For this review, use the dimensioned drawing (mm, ordinates from the lowest corner) and the shaded views. Give positions to 0.01 mm unless a question says otherwise; leave off trailing zeros. Order: outer loops, then holes, each group sorted by start corner. A loop starts at its lowest first (then second) coordinate and runs counter-clockwise, first axis right, second up. Notation, with made-up numbers: (5, 77.5) - (23, 77.5) arc R25 cw to (23, 111.5) - close; hole circle Ø4 at (31.5, 43.5). An arc over 180 degrees is marked (long way). Use a Markdown table: item, result. Add a question column.
1) We need section C-C on z = 16. Write out the cut boundary in (x, y), then the cut area to 3 significant figures.
2) Mouldability with a two-part tool opening along Y and no side actions: class the marked faces 1, 2 and 3 as released by +Y, released by -Y, zero draft, split by the parting line, or undercut.
3) Clearance check with flat-ended pins moving along their axes: P1, Ø3, axis at y = 29, z = 45, coming from the -X side; P2, Ø3, axis at y = 40, z = 16, coming from the -X side; P3, Ø12, axis at x = 164, y = 180, coming from the +Z side. State where each tip first meets the part, or that it passes through.
4) We need section A-A on x = 101.6. Write out the cut boundary in (y, z).
5) We need section B-B on z = 34.5. Write out the cut boundary in (x, y).
6) Wall thickness on L1, parallel to X at y = 101, z = 25; L2, parallel to Y at x = 101.6, z = 28; L3, parallel to X at y = 80, z = 44: over which ranges is each line inside the solid? List them lowest first.
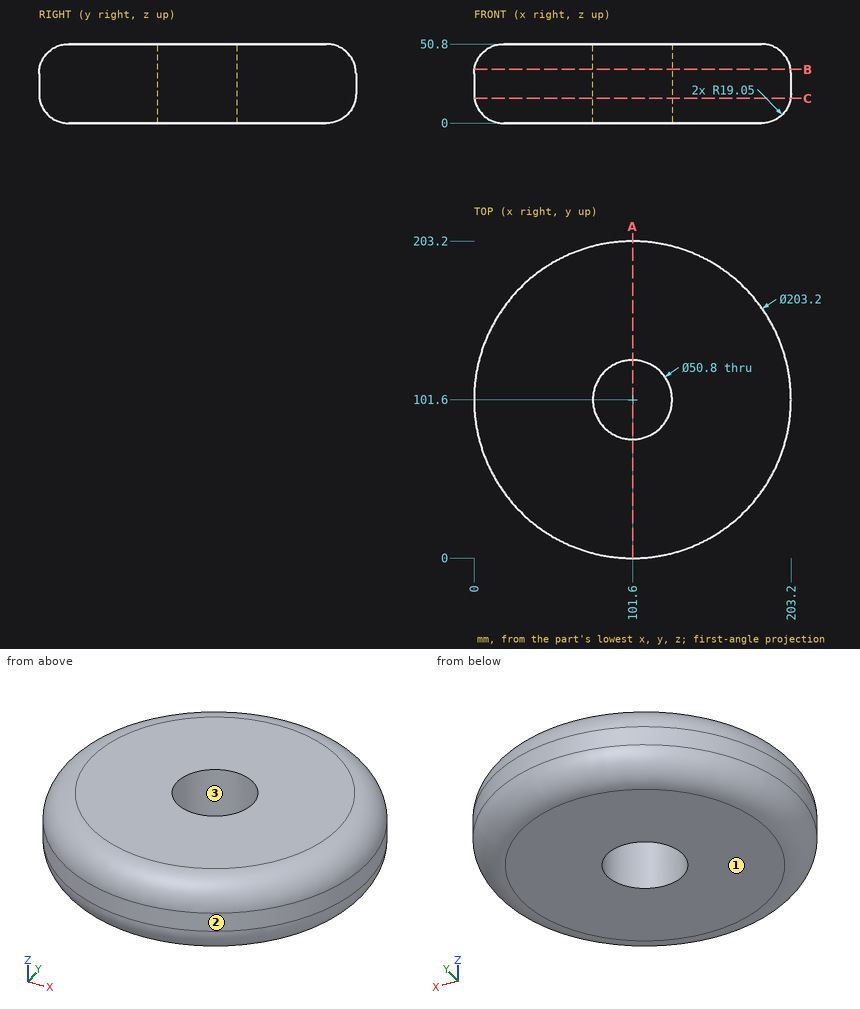
Checked values:
| question | item | result |
|---|---|---|
| 1 | outline | circle Ø202.71 at (101.6, 101.6); hole circle Ø50.8 at (101.6, 101.6) |
| 1 | area | 30,200 mm² |
| 2 | face 1 | zero draft |
| 2 | face 2 | split by the parting line |
| 2 | face 3 | undercut |
| 3 | P1 | x = 35.81 |
| 3 | P2 | x = 19.95 |
| 3 | P3 | z = 46.82 |
| 4 | outline | (0, 19.05) arc R19.05 ccw to (19.05, 0) - (76.2, 0) - (76.2, 50.8) - (19.05, 50.8) arc R19.05 ccw to (0, 31.75) - close; (127, 0) - (184.15, 0) arc R19.05 ccw to (203.2, 19.05) - (203.2, 31.75) arc R19.05 ccw to (184.15, 50.8) - (127, 50.8) - close |
| 5 | outline | circle Ø202.8 at (101.6, 101.6); hole circle Ø50.8 at (101.6, 101.6) |
| 6 | L1 | 0 to 76.21, 126.99 to 203.2 |
| 6 | L2 | 0 to 76.2, 127 to 203.2 |
| 6 | L3 | 6.89 to 88.24, 114.96 to 196.31 |
